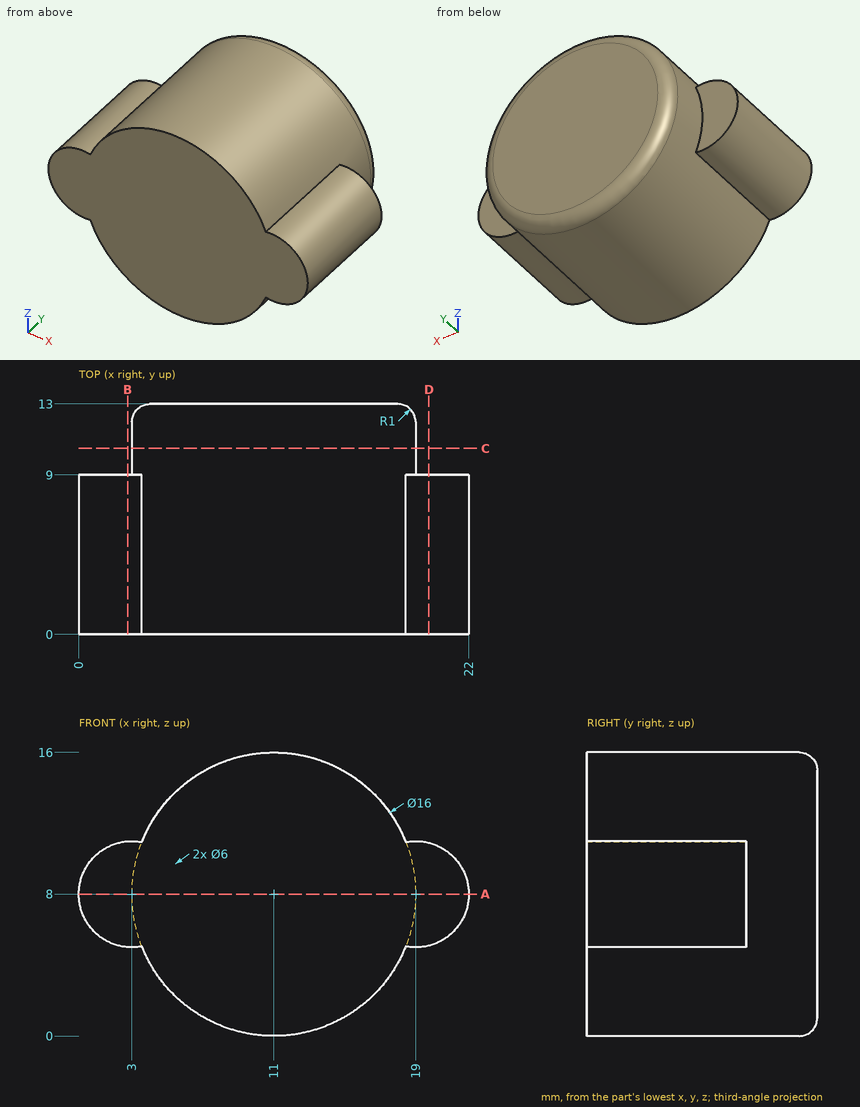
Part print with two shaded views. Sizes in mm from the minimum x, y, z corner. Coordinates: 2 decimals unless noted, no trailing zeros. Write each loop counter-clockwise with the first axis right and the second up, starting at its lowest first coordinate (ties: lowest second). Pieces come first, ordered by that corner, then holes.
(1) Cut at D-D on x = 19.75. List the corners of the cut face in (y, z).
(2) Drill centre lines: line 1 (Z direction, x = 4.75, y = 3.75); line 2 (Z direction, x = 10.75, y = 2); line 3 (X direction, y = 2.5, z = 12). Where is each one in solid material? Low to high.
(3) Cut at A-A on z = 8. List the corners of the cut face in (x, y), and give its area (3 significant figures).
(4) Cut at C-C on y = 10.5. List the corners of the cut face in (x, z).
(5) Cut at B-B on x = 2.75. List the corners of the cut face in (y, z).
(6) Pin check, flat tips, straight feed: pin 1 Ø4 at (y, z) = (2, 11) entering from -X; pin 2 Ø1.1 at (x, z) = (1.5, 9.5) entering from +Y; pin 3 Ø5 at (y, z) = (1.5, 4.5) entering from +X. Stop position of each tip, or through.
Working result:
1. outline: (0, 5.1) - (9, 5.1) - (9, 10.9) - (0, 10.9) - close
2. line 1: z = 3.01 to 12.99
2. line 2: z = 0 to 16
2. line 3: x = 4.07 to 17.93
3. outline: (0, 0) - (22, 0) - (22, 9) - (19, 9) - (19, 12) arc R1 ccw to (18, 13) - (4, 13) arc R1 ccw to (3, 12) - (3, 9) - (0, 9) - close
3. area: 262 mm2
4. outline: circle Ø16 at (11, 8)
5. outline: (0, 5.01) - (9, 5.01) - (9, 10.99) - (0, 10.99) - close
6. pin 1: stops at x = 0.17
6. pin 2: stops at y = 9
6. pin 3: stops at x = 21.83
